Model file for the job. Use its own axes, mm. A direction names the side the tool comes from. Coordinates: 2 decimals unless noted, no trailing zeros. Write each loop counter-clockwise with the first axis right and the second up, starting at its lowest first coordinate (ties: lowest second). Pieces come first, ordered by that corner, then holes. Notation, with made-up numbers: M 8,48 L 41,48 A13 cw 41,52 Z; hole C 58.5,13.25 d7. An arc over 180 degrees is marked long. One line per question, with ' | ' between items. Start each with the question number.
(1) Wall check: probe 1 along Z at (x, y) = (0, 301) (3 decimals); probe 2 along Z at (x, y) = (236.5, 303.5) (3 decimals); probe 3 along X at (y, z) = (300.5, 752). Give the ranges that are in metal, low to high.
(2) Cut at A-A (z = 878.5). Write the cut outline in (x, y), plus the area to 3 significant figures.
(3) Cut at D-D (y = 301.25). Write the cut outline in (x, z) (3 decimals), plus the area to 3 significant figures.
(4) Cut at B-B (x = -104). Write the cut outline in (y, z) (3 decimals).
(5) Two-plate mould, pull along Z, no slides. Class faces 1 (the face through (-4, 304.8, 1141)), 2 (the face through (-1.14, 301.67, 1089.03)): +Z half, -Z half, draft (parallel to the pull), parting line (faces both ways), or undercut.
(6) Tool access for faces 3 (the face through (-4, 298.45, 1141)), 4 (the face through (1.14, 301.67, 739.77)): list every direction of +Z, -Z, +X, -X, +Y, -Y with a clear straight run to the whole face (end or side of a thin tool).
(7) Cut at C-C (x = 0). Write the cut outline in (y, z) (3 decimals).
from build123d import *

# Parameters (mm, degrees)
SKETCH002_W  = 584.2
SKETCH002_H  = 501.65
SKETCH002_R  = 12.7
PAD008_DEPTH = 6.35


with BuildPart() as part:
    # Sketch002 → Pad008 (new body)
    with BuildSketch(Plane(origin=(0, 304.8, 914.4), x_dir=(1, 0, 0), z_dir=(0, -1, 0))):
        Rectangle(SKETCH002_W, SKETCH002_H)
        with Locations((0, 200.025)):
            Circle(SKETCH002_R, mode=Mode.SUBTRACT)
        with Locations((0, -200.025)):
            Circle(SKETCH002_R, mode=Mode.SUBTRACT)
        with BuildLine():
            Line((-241.3, 200.025), (-241.3, -200.025))
            Line((-241.3, -200.025), (-76.2, -200.025))
            ThreePointArc((76.2, -200.025), (0, -174.625), (-76.2, -200.025))
            Line((241.3, -200.025), (76.2, -200.025))
            Line((241.3, 200.025), (241.3, -200.025))
            Line((241.3, 200.025), (76.2, 200.025))
            ThreePointArc((-76.2, 200.025), (0, 174.625), (76.2, 200.025))
            Line((-241.3, 200.025), (-76.2, 200.025))
        make_face(mode=Mode.SUBTRACT)
    extrude(amount=PAD008_DEPTH)


solid = part.part
Filled in:
1) probe 1: 663.575 to 701.675, 727.075 to 739.775, 1089.025 to 1101.725, 1127.125 to 1165.225 | probe 2: 663.575 to 714.375, 1114.425 to 1165.225 | probe 3: -292.1 to -241.3, 241.3 to 292.1
2) outline: M -292.1,298.45 L -241.3,298.45 L -241.3,304.8 L -292.1,304.8 Z; M 241.3,298.45 L 292.1,298.45 L 292.1,304.8 L 241.3,304.8 Z | area: 645 mm²
3) outline: M -292.1,663.575 L 292.1,663.575 L 292.1,1165.225 L -292.1,1165.225 Z; hole M -241.3,714.375 L -76.2,714.375 A127 cw 76.2,714.375 L 241.3,714.375 L 241.3,1114.425 L 76.2,1114.425 A127 cw -76.2,1114.425 L -241.3,1114.425 Z; hole C 0,714.375 d25.4; hole C 0,1114.425 d25.4 | area: 104,000 mm²
4) outline: M 298.45,663.575 L 304.8,663.575 L 304.8,714.375 L 298.45,714.375 Z; M 298.45,1114.425 L 304.8,1114.425 L 304.8,1165.225 L 298.45,1165.225 Z
5) face 1: draft | face 2: undercut
6) face 3: +Z, -Z, +X, -X, -Y | face 4: +Y, -Y
7) outline: M 298.45,663.575 L 304.8,663.575 L 304.8,701.675 L 298.45,701.675 Z; M 298.45,727.075 L 304.8,727.075 L 304.8,739.775 L 298.45,739.775 Z; M 298.45,1089.025 L 304.8,1089.025 L 304.8,1101.725 L 298.45,1101.725 Z; M 298.45,1127.125 L 304.8,1127.125 L 304.8,1165.225 L 298.45,1165.225 Z
